Design review of the part shown in the three views and the two pictorial views. Dimensions are in mm from the part's minimum x, y and z. Round coordinates to 2 decimals unless told otherwise and drop trailing zeros. Loops run counter-clockwise (first coordinate to the right, second up) from the corner with the lowest first, then second, coordinate; pieces in that order, holes last. Notation, with made-up numbers: M 82.5,29.5 L 86.5,29.5 A6 ccw 86.5,39.5 Z; hole C -21,48.25 d2. An arc over 180 degrees is marked long. One line per question, with ' | ' between items. Start each with the question number.
1) We need section A-A (z = 113). Give the boundary of the cut face in (x, y) (3 decimals), and give its area (3 significant figures).
2) We need section C-C (y = 1.6). Give the boundary of the cut face in (x, z) (3 decimals), and give its area (3 significant figures).
3) For pin 1 Ø5 at (x, z) = (57.5, 43.5) entering from -Y, flat-tipped, find the tip position at first contact; note if it passes through.
4) We need section B-B (x = 15). Give the boundary of the cut face in (y, z) (3 decimals), and give its area (3 significant figures).
5) For probe 1 along Z at (x, y) = (26, 2.9); probe 2 along X at (y, z) = (1.55, 69); probe 3 along X at (y, z) = (1.45, 7) (3 decimals), list the stretches that pass through material, from the lowest coordinate up. Write a range as from..to.
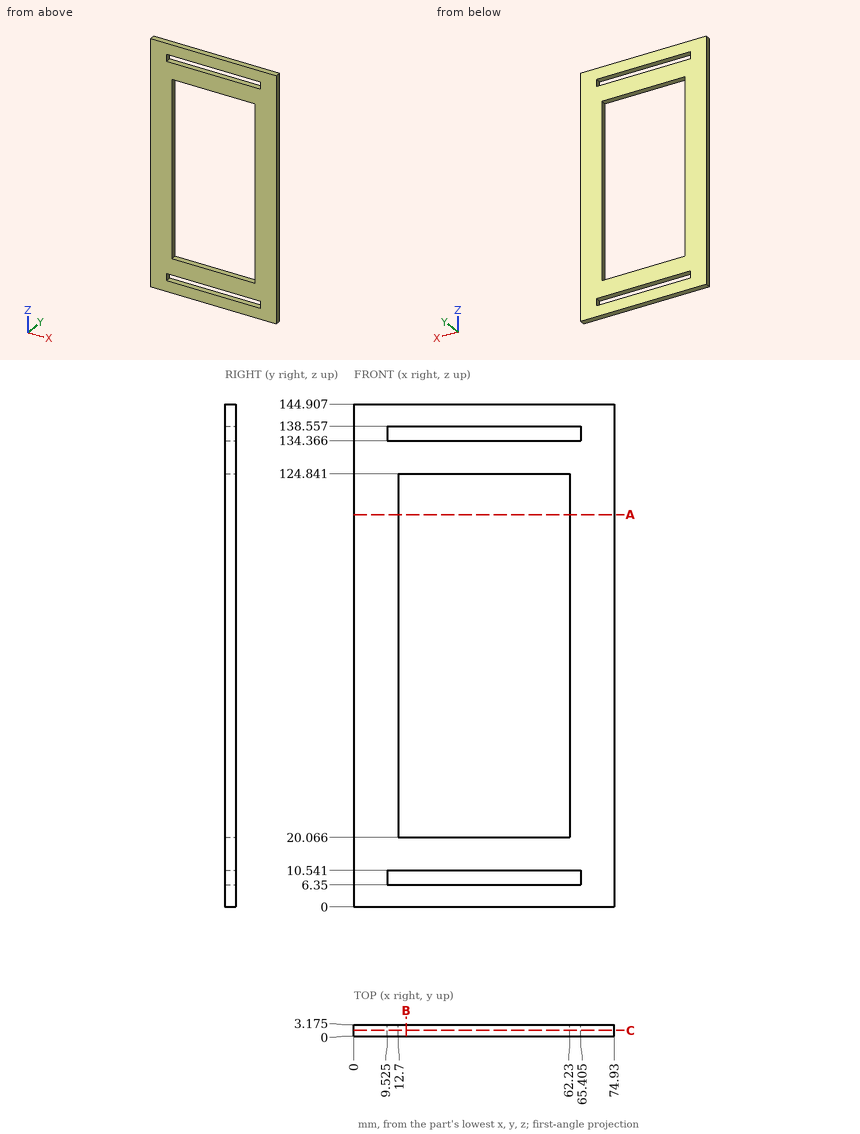
Answers below:
1) outline: M 0,0 L 12.7,0 L 12.7,3.175 L 0,3.175 Z; M 62.23,0 L 74.93,0 L 74.93,3.175 L 62.23,3.175 Z | area: 80.6 mm^2
2) outline: M 0,0 L 74.93,0 L 74.93,144.907 L 0,144.907 Z; hole M 9.525,6.35 L 65.405,6.35 L 65.405,10.541 L 9.525,10.541 Z; hole M 9.525,134.366 L 65.405,134.366 L 65.405,138.557 L 9.525,138.557 Z; hole M 12.7,20.066 L 62.23,20.066 L 62.23,124.841 L 12.7,124.841 Z | area: 5,200 mm^2
3) pin 1: through
4) outline: M 0,0 L 3.175,0 L 3.175,6.35 L 0,6.35 Z; M 0,10.541 L 3.175,10.541 L 3.175,20.066 L 0,20.066 Z; M 0,124.841 L 3.175,124.841 L 3.175,134.366 L 0,134.366 Z; M 0,138.557 L 3.175,138.557 L 3.175,144.907 L 0,144.907 Z | area: 101 mm^2
5) probe 1: 0..6.35, 10.54..20.07, 124.84..134.37, 138.56..144.91 | probe 2: 0..12.7, 62.23..74.93 | probe 3: 0..9.525, 65.405..74.93
